```python
from build123d import *

# Parameters (mm, degrees)
SKETCH1_W           = 30
SKETCH1_H           = 15
BOSS_EXTRUDE1_DEPTH = 150
SKETCH2_R           = 12.7
CUT_EXTRUDE1_DEPTH  = 5
SKETCH3_R           = 9
BOSS_EXTRUDE2_DEPTH = 25
SKETCH4_W           = 150
SKETCH4_H           = 20
BOSS_EXTRUDE3_DEPTH = 150
SKETCH5_R           = 42.5
CUT_EXTRUDE2_DEPTH  = 150
SKETCH6_R           = 60
CUT_EXTRUDE3_DEPTH  = 15
SKETCH7_R           = 2
CUT_EXTRUDE4_DEPTH  = 15
SKETCH17_R          = 2
CUT_EXTRUDE5_DEPTH  = 20
SKETCH18_R          = 2
CUT_EXTRUDE6_DEPTH  = 20


with BuildPart() as part:
    # Sketch1 → Boss-Extrude1 (new body)
    with BuildSketch(Plane(origin=(0, 0, 0), x_dir=(0, 0, -1), z_dir=(1, 0, 0))):
        with Locations((-6.718464351, -7.5)):
            Rectangle(SKETCH1_W, SKETCH1_H)
    extrude(amount=BOSS_EXTRUDE1_DEPTH)

    # Sketch2 → Cut-Extrude1 (cut)
    with BuildSketch(Plane.XZ.offset(15)):
        with Locations(Location((75, 6.718464351, 0), (0, 0, 270))):
            Circle(SKETCH2_R)
    extrude(amount=-CUT_EXTRUDE1_DEPTH, mode=Mode.SUBTRACT)

    # Sketch3 → Boss-Extrude2 (add)
    with BuildSketch(Plane.XZ.offset(10)):
        with Locations(Location((75, 6.718464351, 0), (0, 0, 270))):
            Circle(SKETCH3_R)
    extrude(amount=BOSS_EXTRUDE2_DEPTH)

    # Sketch4 → Boss-Extrude3 (add)
    with BuildSketch(Plane(origin=(0, 0, 0), x_dir=(1, 0, 0), z_dir=(0, 1, 0))):
        with Locations((75, -1.718464351)):
            Rectangle(SKETCH4_W, SKETCH4_H)
    extrude(amount=BOSS_EXTRUDE3_DEPTH)

    # Sketch5 → Cut-Extrude2 (cut)
    with BuildSketch(Plane.XY.offset(11.718464351)):
        with BuildLine():
            Line((75, 150), (0, 150))
            Line((0, 150), (0, 75))
            ThreePointArc((0, 75), (21.966991411, 128.033008589), (75, 150))
        make_face()
        with BuildLine():
            Line((150, 150), (75, 150))
            ThreePointArc((75, 150), (128.033008589, 128.033008589), (150, 75))
            Line((150, 75), (150, 150))
        make_face()
        with Locations((75, 75)):
            Circle(SKETCH5_R)
    extrude(amount=-CUT_EXTRUDE2_DEPTH, mode=Mode.SUBTRACT)

    # Sketch6 → Cut-Extrude3 (cut)
    with BuildSketch(Plane.XY.offset(11.718464351)):
        with Locations((75, 75)):
            Circle(SKETCH6_R)
    extrude(amount=-CUT_EXTRUDE3_DEPTH, mode=Mode.SUBTRACT)

    # Sketch7 → Cut-Extrude4 (cut)
    with BuildSketch(Plane.XY.offset(-3.281535649)):
        with Locations((75, 123)):
            Circle(SKETCH7_R)
        with Locations((108.941125497, 108.941125497)):
            Circle(SKETCH7_R)
        with Locations((123, 75)):
            Circle(SKETCH7_R)
        with Locations((108.941125497, 41.058874503)):
            Circle(SKETCH7_R)
        with Locations((75, 27)):
            Circle(SKETCH7_R)
        with Locations((41.058874503, 41.058874503)):
            Circle(SKETCH7_R)
        with Locations((27, 75)):
            Circle(SKETCH7_R)
        with Locations((41.058874503, 108.941125497)):
            Circle(SKETCH7_R)
    extrude(amount=-CUT_EXTRUDE4_DEPTH, mode=Mode.SUBTRACT)

    # Sketch17 → Cut-Extrude5 (cut)
    with BuildSketch(Plane.XY.offset(11.718464351)):
        with Locations((7.5, 10)):
            Circle(SKETCH17_R)
        with Locations((142.5, 10)):
            Circle(SKETCH17_R)
        with Locations((142.5, 45)):
            Circle(SKETCH17_R)
        with Locations((142.5, 80)):
            Circle(SKETCH17_R)
        with Locations((7.5, 45)):
            Circle(SKETCH17_R)
        with Locations((7.5, 80)):
            Circle(SKETCH17_R)
    extrude(amount=-CUT_EXTRUDE5_DEPTH, mode=Mode.SUBTRACT)

    # Sketch18 → Cut-Extrude6 (cut)
    with BuildSketch(Plane.XY.offset(11.718464351)):
        with Locations((30, 125)):
            Circle(SKETCH18_R)
        with Locations((120, 125)):
            Circle(SKETCH18_R)
    extrude(amount=-CUT_EXTRUDE6_DEPTH, mode=Mode.SUBTRACT)


solid = part.part
```
Verification items for the finished model (mm, model axes). A direction names the side the tool comes from. Round coordinates to 2 decimals unless told otherwise and drop trailing zeros. Write each loop counter-clockwise with the first axis right and the second up, starting at its lowest first coordinate (ties: lowest second). Pieces come first, ordered by that corner, then holes. Notation, with made-up numbers: (61, 62) -> (97, 62) arc R15 cw to (97, 87) -> close; hole circle Ø2 at (10.25, -25.75). An arc over 180 degrees is marked (long way). Write each question's results on one line, items separated by ' | '. Start each with the question number.
1. Material ranges on probe 1 along Y at (x, z) = (75, 3); probe 2 along Z at (x, y) = (40, 50); probe 3 along Y at (x, z) = (47.5, 13), recorded low to high. Write a range as from..to.
2. Cross-section at C-C (y = 53). Enter the section's corners in (x, z).
3. Set-up check for faces 5 (the cylindrical face through (73.35, 149.98, 1.86)), 6 (the flat face through (87, 116, -3.282)), 7 (the cylindrical face through (87.592, -12.535, 8.372)): record each of +Z, -Z, +X, -X, +Y, -Y from which the full face is reachable in a straight line by a thin tool's end or side.
4. Depth check by flat-ended pin: P1, Ø5, axis at x = 75, y = 123, coming from the -Z side; P2, Ø3.5, axis at x = 27, y = 75, coming from the -Z side; P3, Ø10, axis at y = 88, z = 10.5, coming from the -X side; P4, Ø3, axis at x = 37.5, z = 16, coming from the +Y side. Enter the tip coordinate at first touch or a pass-through.
5. Cross-section at D-D (y = 80). Enter the section's corners in (x, z), then the cut area to 3 significant figures.
6. Cross-section at A-A (x = 75). Count the separate pieces of the cut face and the enclosed holes in it, then the cut area to 3 significant figures.
7. Draft check along X on faces 1 (the flat face through (0, 29, 4)), 2 (the flat face through (74, 0, 17)), 3 (the cylindrical face through (140.9, 43.8, 1.9)), 4 (the flat face through (150, 29, 4)). Enter one of: +X half, -X half, draft (parallel to the pull), parting line (faces both ways), or undercut.
8. Cross-section at B-B (y = -13). Enter the section's corners in (x, z).
Solutions:
1) probe 1: y = -35..15, 135..150 | probe 2: z = -8.28..-3.28 | probe 3: y = -15..0
2) outline: (0, -8.28) -> (38.64, -8.28) -> (38.64, -3.28) -> (19.18, -3.28) -> (19.18, 11.72) -> (0, 11.72) -> close; (111.36, -8.28) -> (150, -8.28) -> (150, 11.72) -> (130.82, 11.72) -> (130.82, -3.28) -> (111.36, -3.28) -> close
3) face 5: +Z, -Z, +Y | face 6: +Z | face 7: -Y
4) P1: stops at z = -8.28 | P2: passes through | P3: stops at x = 0.43 | P4: stops at y = 0
5) outline: (0.17, -8.28) -> (5.5, -8.28) -> (5.5, 11.72) -> (0.17, 11.72) -> close; (9.5, -8.28) -> (32.8, -8.28) -> (32.8, -3.28) -> (15.21, -3.28) -> (15.21, 11.72) -> (9.5, 11.72) -> close; (117.2, -8.28) -> (140.5, -8.28) -> (140.5, 11.72) -> (134.79, 11.72) -> (134.79, -3.28) -> (117.2, -3.28) -> close; (144.5, -8.28) -> (149.83, -8.28) -> (149.83, 11.72) -> (144.5, 11.72) -> close | area: 618 mm2
6) separate pieces: 4 | enclosed holes: 0 | area: 1,510 mm2
7) face 1: -X half | face 2: draft | face 3: undercut | face 4: +X half
8) outline: (0, -8.28) -> (150, -8.28) -> (150, 21.72) -> (0, 21.72) -> close; circle Ø18 at (75, 6.72); hole circle Ø25.4 at (75, 6.72)
